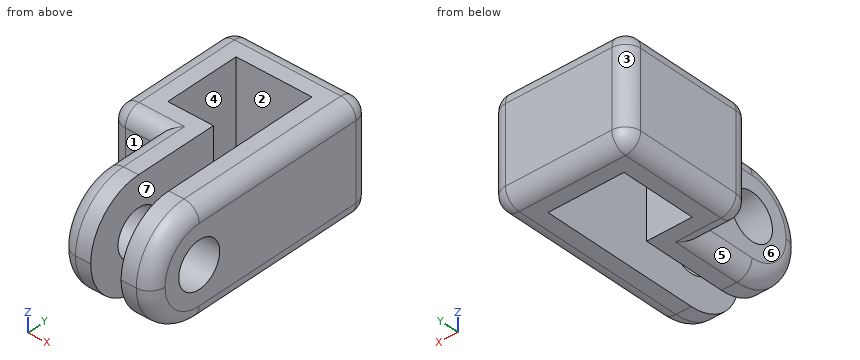
```python
from build123d import *

# Parameters (mm, degrees)
SKETCH_1_W          = 2
SKETCH_1_H          = 7
EXTRUDE_2_DEPTH     = 7
FILLET_4_R          = 3.5
SKETCH_3_R          = 1.5
CUT_EXTRUDE_2_DEPTH = 15.739402973
FILLET_5_R          = 1


with BuildPart() as part:
    # 草图1 → 凸台-拉伸2 (new body)
    with BuildSketch(Plane.XY):
        Polygon((-2.5, -2.5), (-2.5, 2.5), (2.5, 2.5), (2.5, -2.5), (2.5, -4.5), (4.5, -4.5), (4.5, 4.5), (-4.5, 4.5), (-4.5, -4.5), (-1.5, -4.5), (0.5, -4.5), (0.5, -2.5), align=None)
        with Locations((-0.5, -8)):
            Rectangle(SKETCH_1_W, SKETCH_1_H)
        with Locations((3.5, -8)):
            Rectangle(SKETCH_1_W, SKETCH_1_H)
    extrude(amount=EXTRUDE_2_DEPTH)

    # 圆角4
    fillet_4_edges = [part.edges().sort_by_distance(p)[0] for p in [
        (3.5, -11.5, 0),
        (3.5, -11.5, 7),
        (-0.5, -11.5, 0),
        (-0.5, -11.5, 7),
    ]]
    fillet(fillet_4_edges, radius=FILLET_4_R - 0.0001)  # a hair under: the kernel refuses the full size

    # 草图3 → 切除-拉伸2 (cut, through all)
    with BuildSketch(Plane.ZY.offset(1.5)):
        with Locations((3.5, -8)):
            Circle(SKETCH_3_R)
    extrude(amount=-CUT_EXTRUDE_2_DEPTH, mode=Mode.SUBTRACT)

    # 圆角5
    fillet_5_edges = [part.edges().sort_by_distance(p)[0] for p in [
        (-4.5, 0, 0),
        (0, 4.5, 0),
        (4.5, -1.75005, 0),
        (-3, -4.5, 0),
        (-4.5, -4.5, 3.5),
        (-4.5, 4.5, 3.5),
        (4.5, 4.5, 3.5),
        (-3, -4.5, 7),
        (-1.5, -6.25005, 0),
        (4.5, -1.75005, 7),
        (4.5, -10.474903023, 5.974903023),
        (4.5, -10.474903023, 1.025096977),
        (-1.5, -6.25005, 7),
        (-1.5, -10.474903023, 5.974903023),
        (-1.5, -10.474903023, 1.025096977),
        (0, 4.5, 7),
        (-4.5, 0, 7),
    ]]
    fillet(fillet_5_edges, radius=FILLET_5_R)


solid = part.part
```
The model under review builds one solid part; all positions refer to its coordinate system, in mm. Face numbers are marked on the shaded views. A direction names the side the tool comes from. Round coordinates to 2 decimals unless told otherwise and drop trailing zeros. Order: outer loops, then holes, each group sorted by start corner. A loop starts at its lowest first (then second) coordinate and runs counter-clockwise, first axis right, second up. Notation, with made-up numbers: M 64,-31 L 85,-31 A27 cw 85,-3 Z; hole C -2.5,-26 d4. An arc over 180 degrees is marked long. Use a Markdown table: item, result.
1) Wall thickness on line 1 along X through (y, z) = (1, 4.75); line 2 along Y through (x, z) = (3.15, 3.5); line 3 along X through (y, z) = (-7, 6): over which ranges is each line inside the solid? List them lowest first. Write a range as [from, to].
Report:
| item | result |
|---|---|
| line 1 | [-4.5, -2.5], [2.5, 4.5] |
| line 2 | [-11.5, -9.5], [-6.5, 4.5] |
| line 3 | [-1.5, 0.5], [2.5, 4.5] |
2) Insertion check: pin 1 (1.5 mm diameter, centred on x = -3, y = -6, fed in from -Z); pin 2 (1.5 mm diameter, centred on y = -5, z = 2.5, fed in from -X); pin 3 (1.6 mm diameter, centred on x = -2.5, z = 3, fed in from -Y). Each pin has a flat end and moves straight along its axis. Give the tip position at first contact, or say it passes through.
Report:
| item | result |
|---|---|
| pin 1 | through |
| pin 2 | x = -4.16 |
| pin 3 | y = -4.5 |
3) Consider section A-A (x = 0.25). Give the number of separate pieces and of enclosed holes in the cut face, then the cut area to 3 significant figures.
Report:
| item | result |
|---|---|
| separate pieces | 2 |
| enclosed holes | 1 |
| area | 64.2 mm^2 |
4) Tool access review of the marked faces 4, 5, 6 and 7: name each direction out of +Z, -Z, +X, -X, +Y, -Y from which nothing blocks a thin tool from reaching the whole face with its end or side.
Report:
| item | result |
|---|---|
| face 4 | +Z, -Z |
| face 5 | -Z, -X, -Y |
| face 6 | +Z, -Z, -X, -Y |
| face 7 | +Z, -Z, -Y |
5) Consider section B-B (x = -2). Write out the cut boundary in (y, z), then the cut area to 3 significant figures.
Report:
| item | result |
|---|---|
| outline | M -4.5,1 A1 ccw -3.5,0 L -2.5,0 L -2.5,7 L -3.5,7 A1 ccw -4.5,6 Z; M 2.5,0 L 3.5,0 A1 ccw 4.5,1 L 4.5,6 A1 ccw 3.5,7 L 2.5,7 Z |
| area | 27.1 mm^2 |
6) Draft analysis for pull direction Y (two halves, no side actions). For the marked faces 1, 2 and 3, state which applies: released by +Y, released by -Y, zero draft, split by the parting line, or undercut.
Report:
| item | result |
|---|---|
| face 1 | released by -Y |
| face 2 | undercut |
| face 3 | released by +Y |
